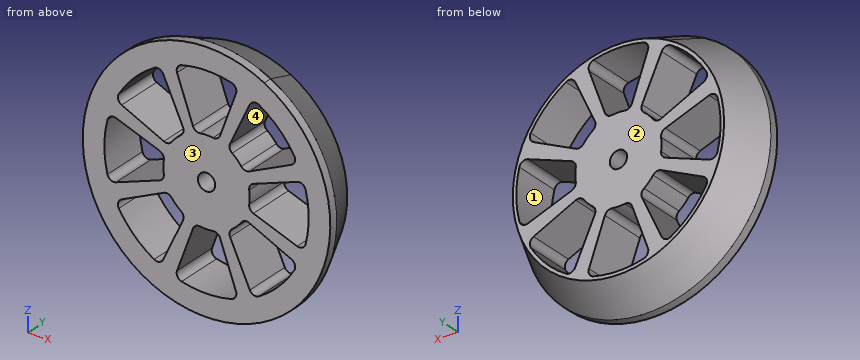
Autodesk Inventor part; units mm, degrees
ref_plane "YZ Plane" through (0, 0, 0) normal (1, 0, 0) x (0, 1, 0)
ref_plane "XZ Plane" through (0, 0, 0) normal (0, 1, 0) x (-1, 0, 0)
ref_plane "XY Plane" through (0, 0, 0) normal (0, 0, 1) x (1, 0, 0)
sketch "Esquisse1" plane through (0, 0, 0) normal (0, 1, 0) x (-1, 0, 0)
  arc A0 (26.7424, 50.7333) -> (-26.7424, 50.7333) centre (0, 0) ccw
  circle A1 centre (0, 0) radius 57.35
  line L0 (0, -80.29) -> (0, 80.29) construction
  line L1 (-80.29, 0) -> (80.29, 0) construction
  circle A2 centre (0, 0) radius 4
  line L2 (-6.2691, 21.7137) -> (-13.6461, 41.982)
  line L3 (13.6461, 41.982) -> (6.2691, 21.7137)
  arc A3 (11.5595, 45.9173) -> (-11.5595, 45.9173) centre (0, 0) ccw
  arc A4 (-11.5595, 45.9173) -> (-13.6461, 41.982) centre (-10.8271, 43.0081) ccw
  arc A5 (13.6461, 41.982) -> (11.5595, 45.9173) centre (10.8271, 43.0081) ccw
  circle A6 centre (0, 0) radius 16 construction
  circle A7 centre (0, 0) radius 57.35 construction
  arc A8 (3, 19.7737) -> (-3, 19.7737) centre (0, 0) ccw
  arc A9 (-6.2691, 21.7137) -> (-3, 19.7737) centre (-3.45, 22.7398) ccw
  arc A10 (3, 19.7737) -> (6.2691, 21.7137) centre (3.45, 22.7398) ccw
  line L4 (-19.7868, 10.921) -> (-39.3351, 20.0365)
  line L5 (-20.0365, 39.3351) -> (-10.921, 19.7868)
  arc A11 (-24.2947, 40.6422) -> (-40.6422, 24.2947) centre (0, 0) ccw
  arc A12 (-40.6422, 24.2947) -> (-39.3351, 20.0365) centre (-38.0672, 22.7554) ccw
  arc A13 (-20.0365, 39.3351) -> (-24.2947, 40.6422) centre (-22.7554, 38.0672) ccw
  arc A14 (-11.8608, 16.1035) -> (-16.1035, 11.8608) centre (0, 0) ccw
  arc A15 (-19.7868, 10.921) -> (-16.1035, 11.8608) centre (-18.519, 13.6399) ccw
  arc A16 (-11.8608, 16.1035) -> (-10.921, 19.7868) centre (-13.6399, 18.519) ccw
  line L6 (-21.7137, -6.2691) -> (-41.982, -13.6461)
  line L7 (-41.982, 13.6461) -> (-21.7137, 6.2691)
  arc A17 (-45.9173, 11.5595) -> (-45.9173, -11.5595) centre (0, 0) ccw
  arc A18 (-45.9173, -11.5595) -> (-41.982, -13.6461) centre (-43.0081, -10.8271) ccw
  arc A19 (-41.982, 13.6461) -> (-45.9173, 11.5595) centre (-43.0081, 10.8271) ccw
  arc A20 (-19.7737, 3) -> (-19.7737, -3) centre (0, 0) ccw
  arc A21 (-21.7137, -6.2691) -> (-19.7737, -3) centre (-22.7398, -3.45) ccw
  arc A22 (-19.7737, 3) -> (-21.7137, 6.2691) centre (-22.7398, 3.45) ccw
  line L8 (-10.921, -19.7868) -> (-20.0365, -39.3351)
  line L9 (-39.3351, -20.0365) -> (-19.7868, -10.921)
  arc A23 (-40.6422, -24.2947) -> (-24.2947, -40.6422) centre (0, 0) ccw
  arc A24 (-24.2947, -40.6422) -> (-20.0365, -39.3351) centre (-22.7554, -38.0672) ccw
  arc A25 (-39.3351, -20.0365) -> (-40.6422, -24.2947) centre (-38.0672, -22.7554) ccw
  arc A26 (-16.1035, -11.8608) -> (-11.8608, -16.1035) centre (0, 0) ccw
  arc A27 (-10.921, -19.7868) -> (-11.8608, -16.1035) centre (-13.6399, -18.519) ccw
  arc A28 (-16.1035, -11.8608) -> (-19.7868, -10.921) centre (-18.519, -13.6399) ccw
  line L10 (6.2691, -21.7137) -> (13.6461, -41.982)
  line L11 (-13.6461, -41.982) -> (-6.2691, -21.7137)
  arc A29 (-11.5595, -45.9173) -> (11.5595, -45.9173) centre (0, 0) ccw
  arc A30 (11.5595, -45.9173) -> (13.6461, -41.982) centre (10.8271, -43.0081) ccw
  arc A31 (-13.6461, -41.982) -> (-11.5595, -45.9173) centre (-10.8271, -43.0081) ccw
  arc A32 (-3, -19.7737) -> (3, -19.7737) centre (0, 0) ccw
  arc A33 (6.2691, -21.7137) -> (3, -19.7737) centre (3.45, -22.7398) ccw
  arc A34 (-3, -19.7737) -> (-6.2691, -21.7137) centre (-3.45, -22.7398) ccw
  line L12 (19.7868, -10.921) -> (39.3351, -20.0365)
  line L13 (20.0365, -39.3351) -> (10.921, -19.7868)
  arc A35 (24.2947, -40.6422) -> (40.6422, -24.2947) centre (0, 0) ccw
  arc A36 (40.6422, -24.2947) -> (39.3351, -20.0365) centre (38.0672, -22.7554) ccw
  arc A37 (20.0365, -39.3351) -> (24.2947, -40.6422) centre (22.7554, -38.0672) ccw
  arc A38 (11.8608, -16.1035) -> (16.1035, -11.8608) centre (0, 0) ccw
  arc A39 (19.7868, -10.921) -> (16.1035, -11.8608) centre (18.519, -13.6399) ccw
  arc A40 (11.8608, -16.1035) -> (10.921, -19.7868) centre (13.6399, -18.519) ccw
  line L14 (21.7137, 6.2691) -> (41.982, 13.6461)
  line L15 (41.982, -13.6461) -> (21.7137, -6.2691)
  arc A41 (45.9173, -11.5595) -> (45.9173, 11.5595) centre (0, 0) ccw
  arc A42 (45.9173, 11.5595) -> (41.982, 13.6461) centre (43.0081, 10.8271) ccw
  arc A43 (41.982, -13.6461) -> (45.9173, -11.5595) centre (43.0081, -10.8271) ccw
  arc A44 (19.7737, -3) -> (19.7737, 3) centre (0, 0) ccw
  arc A45 (21.7137, 6.2691) -> (19.7737, 3) centre (22.7398, 3.45) ccw
  arc A46 (19.7737, -3) -> (21.7137, -6.2691) centre (22.7398, -3.45) ccw
  line L16 (10.921, 19.7868) -> (20.0365, 39.3351)
  line L17 (39.3351, 20.0365) -> (19.7868, 10.921)
  arc A47 (40.6422, 24.2947) -> (24.2947, 40.6422) centre (0, 0) ccw
  arc A48 (24.2947, 40.6422) -> (20.0365, 39.3351) centre (22.7554, 38.0672) ccw
  arc A49 (39.3351, 20.0365) -> (40.6422, 24.2947) centre (38.0672, 22.7554) ccw
  arc A50 (16.1035, 11.8608) -> (11.8608, 16.1035) centre (0, 0) ccw
  arc A51 (10.921, 19.7868) -> (11.8608, 16.1035) centre (13.6399, 18.519) ccw
  arc A52 (16.1035, 11.8608) -> (19.7868, 10.921) centre (18.519, 13.6399) ccw
  point P0 (0, 0)
  point P1 (-14.7432, 44.9962)
  point P2 (14.7432, 44.9962)
  point P3 (5.3773, 19.2636)
  point P4 (-5.3773, 19.2636)
  point P5 (-42.2422, 21.3921)
  point P6 (-21.3921, 42.2422)
  point P7 (-9.8191, 17.4237)
  point P8 (-17.4237, 9.8191)
  point P9 (-44.9962, -14.7432)
  point P10 (-44.9962, 14.7432)
  point P11 (-19.2636, 5.3773)
  point P12 (-19.2636, -5.3773)
  point P13 (-21.3921, -42.2422)
  point P14 (-42.2422, -21.3921)
  point P15 (-17.4237, -9.8191)
  point P16 (-9.8191, -17.4237)
  point P17 (14.7432, -44.9962)
  point P18 (-14.7432, -44.9962)
  point P19 (-5.3773, -19.2636)
  point P20 (5.3773, -19.2636)
  point P21 (42.2422, -21.3921)
  point P22 (21.3921, -42.2422)
  point P23 (9.8191, -17.4237)
  point P24 (17.4237, -9.8191)
  point P25 (44.9962, 14.7432)
  point P26 (44.9962, -14.7432)
  point P27 (19.2636, -5.3773)
  point P28 (19.2636, 5.3773)
  point P29 (21.3921, 42.2422)
  point P30 (42.2422, 21.3921)
  point P31 (17.4237, 9.8191)
  point P32 (9.8191, 17.4237)
  dimension "d0" = 8
  dimension "d2" = 3
  dimension "d3" = 10
  dimension "d5" = 40
  dimension "d15" = 20
  dimension "d16" = 3
  dimension "d17" = 6
  dimension "d20" = 360
extrude "Extrusion1" add sketch "Esquisse1" against normal blind 22
chamfer "Chanfrein1" distance 18 angle 25 1 edges at (57.35, 0, 0) measured on face at (-31.6781, -14.6667, -47.8071)
properties part number "Colossus_7kW_Rotor"
Here's how the part is built. I have some questions about the finished solid (model axes, mm). Face numbers are marked on the shaded views. A direction names the side the tool comes from. Coordinates: 2 decimals unless noted, no trailing zeros. Order: outer loops, then holes, each group sorted by start corner. A loop starts at its lowest first (then second) coordinate and runs counter-clockwise, first axis right, second up.
Item 1: Thinking about a two-plate mould opening in Z: for the marked faces 3 and 4, which applies, pulls with the +Z half, pulls with the -Z half, needs draft (parallel to the pull), parting line crosses it, or undercut?
Response values:
face 3: needs draft
face 4: undercut
Item 2: If we section it at B-B, the plane x = 0: List the corners of the cut face in (y, z) for me.
Response values:
outline: (-22, -57.35) - (-18, -57.35) - (0, -48.96) - (0, -47.35) - (-22, -47.35) - close; (-22, -20) - (0, -20) - (0, -4) - (-22, -4) - close; (-22, 4) - (0, 4) - (0, 20) - (-22, 20) - close; (-22, 47.35) - (0, 47.35) - (0, 48.96) - (-18, 57.35) - (-22, 57.35) - close
Item 3: Which directions (+Z, -Z, +X, -X, +Y, -Y) give clear straight access to the entire face, cutting with the end or side of a thin tool? Please do the marked faces 1 and 2.
Response values:
face 1: +Y, -Y
face 2: +Z, -Z, +X, -X, +Y
Item 4: If we section it at C-C, the plane y = -19.75: Give the number of separate pieces and of enclosed holes in the cut face, then the cut area to 3 significant figures.
Response values:
separate pieces: 1
enclosed holes: 9
area: 5,870 mm2
Item 5: I'm going to push flat-ended pins straight in: pin 1 Ø2 at (y, z) = (-18, 3) entering from -X; pin 2 Ø8 at (x, z) = (19, -12) entering from -Y; pin 3 Ø3 at (x, y) = (17.5, -6.5) entering from +Z; pin 4 Ø1 at (y, z) = (-5, 22) entering from +X. Where does each tip first touch, or does it pass through?
Response values:
pin 1: stops at x = -57.32
pin 2: stops at y = -22
pin 3: stops at z = 49.86
pin 4: stops at x = 46.68
Item 6: If we section it at A-A, the plane z = 0: List the corners of the cut face in (x, y) for me.
Response values:
outline: (-57.35, -22) - (-47.35, -22) - (-47.35, 0) - (-48.96, 0) - (-57.35, -18) - close; (-20, -22) - (-4, -22) - (-4, 0) - (-20, 0) - close; (4, -22) - (20, -22) - (20, 0) - (4, 0) - close; (47.35, -22) - (57.35, -22) - (57.35, -18) - (48.96, 0) - (47.35, 0) - close
Item 7: I need wall thicknesses on probe 1 along Z at (x, y) = (0, -8.5); probe 2 along X at (y, z) = (-18.5, 14.5); probe 3 along X at (y, z) = (-5.25, -2.5). Which ranges of each line are inside material? Lowest first, please.
Response values:
probe 1: z = -52.92 to -47.35, -20 to -4, 4 to 20, 47.35 to 52.92
probe 2: x = -55.49 to -27.46, -13.78 to 13.78, 27.46 to 55.49
probe 3: x = -51.34 to -47.28, -19.84 to -3.12, 3.12 to 19.84, 47.28 to 51.34
